Verification items for the finished model (mm, model axes). Give positions to 0.01 mm unless a question says otherwise; leave off trailing zeros. Order: outer loops, then holes, each group sorted by start corner. A loop starts at its lowest first (then second) coordinate and runs counter-clockwise, first axis right, second up.
from build123d import *

# Parameters (mm, degrees)
SKETCH1_W           = 92.964
SKETCH1_H           = 38.1
SKETCH1_R           = 1.651
BOSS_EXTRUDE1_DEPTH = 3.175
SKETCH2_W           = 74.041
SKETCH2_H           = 21.59
CUT_EXTRUDE1_DEPTH  = 3.175


with BuildPart() as part:
    # Sketch1 → Boss-Extrude1 (new body)
    with BuildSketch(Plane(origin=(0, 0, 0), x_dir=(1, 0, 0), z_dir=(0, 1, 0))):
        Rectangle(SKETCH1_W, SKETCH1_H)
        with Locations(Location((-35.567692741, -15.875, 0), (0, 0, 270))):
            Circle(SKETCH1_R, mode=Mode.SUBTRACT)
        with Locations(Location((-35.567692741, 15.875, 0), (0, 0, 270))):
            Circle(SKETCH1_R, mode=Mode.SUBTRACT)
        with Locations(Location((40.132, 15.875, 0), (0, 0, 270))):
            Circle(SKETCH1_R, mode=Mode.SUBTRACT)
        with Locations(Location((40.132, -15.875, 0), (0, 0, 270))):
            Circle(SKETCH1_R, mode=Mode.SUBTRACT)
        with Locations(Location((-35.567692741, 0, 0), (0, 0, 270))):
            Circle(SKETCH1_R, mode=Mode.SUBTRACT)
    extrude(amount=BOSS_EXTRUDE1_DEPTH)

    # Sketch2 → Cut-Extrude1 (cut)
    with BuildSketch(Plane(origin=(0, 3.175, 0), x_dir=(1, 0, 0), z_dir=(0, 1, 0))):
        with Locations((9.4615, 0)):
            Rectangle(SKETCH2_W, SKETCH2_H)
    extrude(amount=-CUT_EXTRUDE1_DEPTH, mode=Mode.SUBTRACT)


solid = part.part
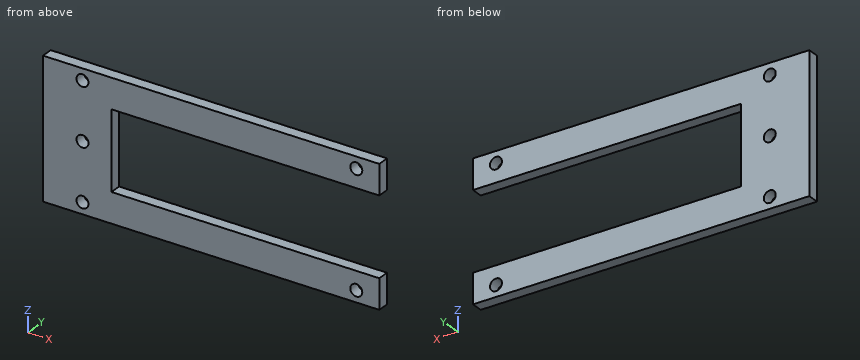
(1) Section check D-D, the plane z = -16. Enter the section's corners in (x, y) (3 decimals), then the cut area to 3 significant figures.
Solved:
outline: (-46.482, 0) - (-37.214, 0) - (-37.214, 3.175) - (-46.482, 3.175) - close; (-33.921, 0) - (38.486, 0) - (38.486, 3.175) - (-33.921, 3.175) - close; (41.778, 0) - (46.482, 0) - (46.482, 3.175) - (41.778, 3.175) - close
area: 274 mm2
(2) Section check A-A, the plane z = 0. Enter the section's corners in (x, y) (3 decimals), then the cut area to 3 significant figures.
Solved:
outline: (-46.482, 0) - (-37.219, 0) - (-37.219, 3.175) - (-46.482, 3.175) - close; (-33.917, 0) - (-27.559, 0) - (-27.559, 3.175) - (-33.917, 3.175) - close
area: 49.6 mm2
(3) Scan lines: line 1 (X direction, y = 2.5, z = 16); line 2 (Z direction, x = 40, y = 1.1) (3 decimals); line 3 (Z direction, x = -22, y = 1.9) (3 decimals). Record each from-to range of solid material in increasing order.
Solved:
line 1: x = -46.48 to -37.21, -33.92 to 38.49, 41.78 to 46.48
line 2: z = -19.05 to -17.521, -14.229 to -10.795, 10.795 to 14.229, 17.521 to 19.05
line 3: z = -19.05 to -10.795, 10.795 to 19.05
(4) Section check C-C, the plane y = 0.9. Enter the section's corners in (x, z) (3 decimals), then the cut area to 3 significant figures.
Solved:
outline: (-46.482, -19.05) - (46.482, -19.05) - (46.482, -10.795) - (-27.559, -10.795) - (-27.559, 10.795) - (46.482, 10.795) - (46.482, 19.05) - (-46.482, 19.05) - close; hole circle Ø3.302 at (-35.568, -15.875); hole circle Ø3.302 at (-35.568, 0); hole circle Ø3.302 at (-35.568, 15.875); hole circle Ø3.302 at (40.132, -15.875); hole circle Ø3.302 at (40.132, 15.875)
area: 1,900 mm2
(5) Section check B-B, the plane x = 2.5. Enter the section's corners in (y, z) (3 decimals), then the cut area to 3 significant figures.
Solved:
outline: (0, -19.05) - (3.175, -19.05) - (3.175, -10.795) - (0, -10.795) - close; (0, 10.795) - (3.175, 10.795) - (3.175, 19.05) - (0, 19.05) - close
area: 52.4 mm2
